For this review, take the finished solid that the model builds, in its own axes (mm). Face numbers are marked on the shaded views. A direction names the side the tool comes from. Coordinates: 2 decimals unless noted, no trailing zeros. Write each loop counter-clockwise with the first axis right and the second up, starting at its lowest first coordinate (ties: lowest second). Pieces come first, ordered by that corner, then holes. Notation, with made-up numbers: (-25.75, 6) -> (-1.75, 6) arc R36 ccw to (-1.75, 43) -> close; hole circle Ø9 at (-25, 70.5). An arc over 180 degrees is marked (long way). One line per item, written item: value. Start each with the question number.
1) For pin 1 Ø12 at (y, z) = (5, -8.5) entering from +X; pin 2 Ø6.5 at (x, y) = (79.5, 2) entering from +Z; pin 3 Ø6 at (x, y) = (64, 7.5) entering from +Z, all flat-tipped, find the tip position at first contact; note any pin that passes through.
2) Add section D-D (y = 19). State the section outline as (x, z) points, and give its area (3 significant figures).
3) Add section B-B (z = -25). State the section outline as (x, y) points, and give its area (3 significant figures).
4) Add section C-C (y = 13). State the section outline as (x, z) points, and give its area (3 significant figures).
5) Add section A-A (x = 46). State the section outline as (y, z) points, and give its area (3 significant figures).
6) Mouldability with a two-part tool opening along X and no side actions: class the marked faces 6, 7 and 8 as released by +X, released by -X, zero draft, split by the parting line, or undercut.
7) For probe 1 along X at (y, z) = (8.5, -25); probe 2 along Y at (x, z) = (44, -32); probe 3 along X at (y, z) = (-0.5, -14), list the stretches that pass through material, from the lowest coordinate up. Write a range as from..to.
8) Machinability: for the marked faces 1, 2, 3, 4 and 5, which of the approach directions +Z, -Z, +X, -X, +Y, -Y give a long, thin tool a straight path to every point of the face, cutting with its end or side? Answer none if there is none.
from build123d import *

# Parameters (mm, degrees)
BOSS_EXTRUDE1_DEPTH  = 4
CUT_EXTRUDE1_DEPTH   = 3
SKETCH5_W            = 49
SKETCH5_H            = 16
BOSS_EXTRUDE2_DEPTH  = 4
BOSS_EXTRUDE15_DEPTH = 30
SKETCH20_R           = 2.4
CUT_EXTRUDE26_DEPTH  = 1
FILLET8_R            = 4
FILLET12_R           = 4
CUT_EXTRUDE_8_DEPTH  = 28
SKETCH_6_R           = 1.05
CUT_EXTRUDE_9_DEPTH  = 20
SKETCH_8_W           = 6
SKETCH_8_H           = 10
CUT_EXTRUDE_10_DEPTH = 8


with BuildPart() as part:
    # Sketch2 → Boss-Extrude1 (new body)
    with BuildSketch(Plane.XY):
        with BuildLine():
            Line((23.733047461, 11.63962887), (23.733047461, -4.36037113))
            Line((23.733047461, -4.36037113), (-21.266952539, -4.36037113))
            ThreePointArc((-21.266952539, -4.36037113), (-27.597931628, 3.63962887), (-21.266952539, 11.63962887))
            Line((-21.266952539, 11.63962887), (23.733047461, 11.63962887))
        make_face()
    extrude(amount=BOSS_EXTRUDE1_DEPTH)

    # Sketch1 → Cut-Extrude1 (cut)
    with BuildSketch(Plane.XY):
        with BuildLine():
            Line((-6.25004119, 8.63962887), (-20.04279291, 6.23962887))
            ThreePointArc((-20.04279291, 6.23962887), (-22.105421524, 3.63962887), (-20.04279291, 1.03962887))
            Line((-20.04279291, 1.03962887), (-6.25004119, -1.36037113))
            ThreePointArc((-6.25004119, -1.36037113), (-2.105421524, -2.86037113), (2.039198142, -1.36037113))
            Line((2.039198142, -1.36037113), (15.831949862, 1.03962887))
            ThreePointArc((15.831949862, 1.03962887), (17.894578476, 3.63962887), (15.831949862, 6.23962887))
            Line((15.831949862, 6.23962887), (2.039198142, 8.63962887))
            ThreePointArc((2.039198142, 8.63962887), (-2.105421524, 10.13962887), (-6.25004119, 8.63962887))
        make_face()
    extrude(amount=CUT_EXTRUDE1_DEPTH, mode=Mode.SUBTRACT)

    # Sketch5 → Boss-Extrude2 (add)
    with BuildSketch(Plane(origin=(23.733047461, 0, 0), x_dir=(0, 0, -1), z_dir=(1, 0, 0))):
        with Locations((20.5, 3.63962887)):
            Rectangle(SKETCH5_W, SKETCH5_H)
    extrude(amount=BOSS_EXTRUDE2_DEPTH)

    # Sketch6 → Boss-Extrude15 (add)
    with BuildSketch(Plane(origin=(0, 0, -45), x_dir=(-1, 0, 0), z_dir=(0, 0, -1))):
        Polygon((-30.946192459, -15.36037113), (-83.733047461, -15.36037113), (-83.733047461, 22.63962887), (-23.733047461, 22.63962887), (-23.733047461, -15.36037113), align=None)
    extrude(amount=-BOSS_EXTRUDE15_DEPTH)

    # Sketch20 → Cut-Extrude26 (cut)
    with BuildSketch(Plane(origin=(0, 0, 3), x_dir=(-1, 0, 0), z_dir=(0, 0, -1))):
        with Locations((2.105421524, 3.63962887)):
            Circle(SKETCH20_R)
    extrude(amount=-CUT_EXTRUDE26_DEPTH, mode=Mode.SUBTRACT)

    # Fillet8
    fillet8_edges = [part.edges().sort_by_distance(p)[0] for p in [
        (23.733047461, 3.63962887, 0),
    ]]
    fillet(fillet8_edges, radius=FILLET8_R)

    # Fillet12
    fillet12_edges = [part.edges().sort_by_distance(p)[0] for p in [
        (27.733047461, 3.63962887, 4),
    ]]
    fillet(fillet12_edges, radius=FILLET12_R)

    # 草圖5 → 除料-伸長8 (cut)
    with BuildSketch(Plane.XY.offset(-15)):
        Polygon((75.733047461, -7.806095257), (75.733047461, 14.193904743), (33.733047461, 14.193904743), (33.733047461, 3.193904743), (33.733047461, -7.806095257), align=None)
    extrude(amount=-CUT_EXTRUDE_8_DEPTH, mode=Mode.SUBTRACT)

    # 草圖6 → 除料-伸長9 (cut)
    with BuildSketch(Plane.XY.offset(-15)):
        with Locations((29.733047461, 8.63962887)):
            Circle(SKETCH_6_R)
        with Locations((29.733047461, -1.36037113)):
            Circle(SKETCH_6_R)
        with Locations((79.733047461, 8.63962887)):
            Circle(SKETCH_6_R)
        with Locations((79.733047461, -1.36037113)):
            Circle(SKETCH_6_R)
    extrude(amount=-CUT_EXTRUDE_9_DEPTH, mode=Mode.SUBTRACT)

    # 草圖8 → 除料-伸長10 (cut)
    with BuildSketch(Plane(origin=(83.733047461, 0, 0), x_dir=(0, 0, -1), z_dir=(1, 0, 0))):
        with Locations((39, 3.238584995)):
            Rectangle(SKETCH_8_W, SKETCH_8_H)
    extrude(amount=-CUT_EXTRUDE_10_DEPTH, mode=Mode.SUBTRACT)


solid = part.part
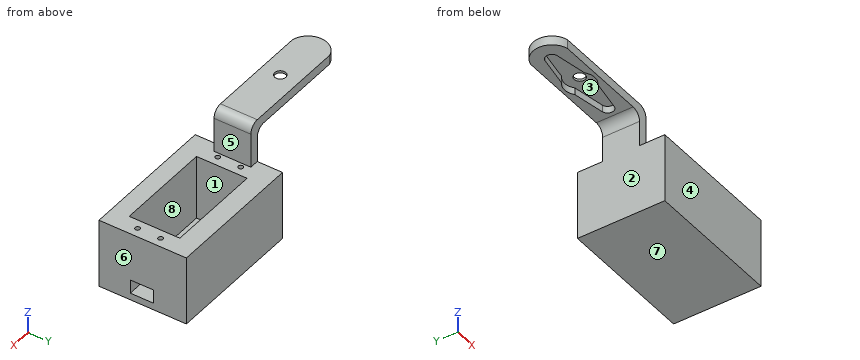
Numbers:
1. pin 1: x = 27.73
1. pin 2: z = -15
1. pin 3: z = -43
2. outline: (23.73, -45) -> (83.73, -45) -> (83.73, -15) -> (23.73, -15) -> close
2. area: 1,800 mm²
3. outline: (23.73, -15.36) -> (83.73, -15.36) -> (83.73, 22.64) -> (23.73, 22.64) -> close; hole circle Ø2.1 at (29.73, -1.36); hole circle Ø2.1 at (29.73, 8.64); hole (33.73, -7.81) -> (75.73, -7.81) -> (75.73, 14.19) -> (33.73, 14.19) -> close; hole circle Ø2.1 at (79.73, -1.36); hole circle Ø2.1 at (79.73, 8.64)
3. area: 1,340 mm²
4. outline: (23.73, -45) -> (83.73, -45) -> (83.73, -15) -> (75.73, -15) -> (75.73, -43) -> (33.73, -43) -> (33.73, -15) -> (23.73, -15) -> close
4. area: 624 mm²
5. outline: (-15.36, -45) -> (22.64, -45) -> (22.64, -15) -> (14.19, -15) -> (14.19, -43) -> (-7.81, -43) -> (-7.81, -15) -> (-15.36, -15) -> close
5. area: 524 mm²
6. face 6: released by +X
6. face 7: zero draft
6. face 8: undercut
7. probe 1: 23.73..28.69, 30.77..33.73, 75.73..78.69, 80.77..83.73
7. probe 2: -15.36..-7.81, 14.19..22.64
7. probe 3: 23.73..27.73
8. face 1: +Z
8. face 2: -Z, -X, +Y, -Y
8. face 3: -Z
8. face 4: +Z, -Z, +X, -X, -Y
8. face 5: +Z, +X, +Y, -Y
